```python
from build123d import *

# Parameters (mm, degrees)
SKETCH1_R           = 1.75
SKETCH1_R_2         = 5
BOSS_EXTRUDE1_DEPTH = 6
SKETCH2_R           = 3
SKETCH2_R_2         = 1.75
CUT_EXTRUDE1_DEPTH  = 3
CUT_EXTRUDE2_START  = -3
SKETCH3_R           = 8
SKETCH3_R_2         = 5
CUT_EXTRUDE2_DEPTH  = 3


with BuildPart() as part:
    # Sketch1 → Boss-Extrude1 (new body)
    with BuildSketch(Plane(origin=(0, 0, 0), x_dir=(1, 0, 0), z_dir=(0, 1, 0))):
        with BuildLine():
            Line((23.69, 13.5), (-31.1, 13.5))
            Line((-31.1, 13.5), (-31.1, 10.5))
            ThreePointArc((-31.1, 10.5), (-20.6, 0), (-31.1, -10.5))
            Line((-31.1, -10.5), (-31.1, -13.5))
            Line((-31.1, -13.5), (23.69, -13.5))
            Line((23.69, -13.5), (23.69, -11))
            ThreePointArc((23.69, -11), (34.69, 0), (23.69, 11))
            Line((23.69, 11), (23.69, 13.5))
        make_face()
        with Locations(Location((-12, -9, 0), (0, 0, 270))):
            Circle(SKETCH1_R, mode=Mode.SUBTRACT)
        with Locations(Location((12, -9, 0), (0, 0, 270))):
            Circle(SKETCH1_R, mode=Mode.SUBTRACT)
        with Locations(Location((-12, 9, 0), (0, 0, 270))):
            Circle(SKETCH1_R, mode=Mode.SUBTRACT)
        with Locations(Location((0, 0, 0), (0, 0, 270))):
            Circle(SKETCH1_R_2, mode=Mode.SUBTRACT)
        with Locations(Location((12, 9, 0), (0, 0, 270))):
            Circle(SKETCH1_R, mode=Mode.SUBTRACT)
        with Locations(Location((23.69, 0, 0), (0, 0, 270))):
            Circle(SKETCH1_R_2, mode=Mode.SUBTRACT)
    extrude(amount=BOSS_EXTRUDE1_DEPTH)

    # Sketch2 → Cut-Extrude1 (cut)
    # profile 1 of 4: a face of its own
    with BuildSketch(Plane.XZ):
        with Locations(Location((-12, -9, 0), (0, 0, 270))):
            Circle(SKETCH2_R)
        with Locations(Location((-12, -9, 0), (0, 0, 270))):
            Circle(SKETCH2_R_2, mode=Mode.SUBTRACT)
    # profile 2 of 4: a face of its own
    with BuildSketch(Plane.XZ):
        with Locations(Location((-12, 9, 0), (0, 0, 270))):
            Circle(SKETCH2_R)
        with Locations(Location((-12, 9, 0), (0, 0, 270))):
            Circle(SKETCH2_R_2, mode=Mode.SUBTRACT)
    # profile 3 of 4: a face of its own
    with BuildSketch(Plane.XZ):
        with Locations(Location((12, 9, 0), (0, 0, 270))):
            Circle(SKETCH2_R)
        with Locations(Location((12, 9, 0), (0, 0, 270))):
            Circle(SKETCH2_R_2, mode=Mode.SUBTRACT)
    # profile 4 of 4: a face of its own
    with BuildSketch(Plane.XZ):
        with Locations(Location((12, -9, 0), (0, 0, 270))):
            Circle(SKETCH2_R)
        with Locations(Location((12, -9, 0), (0, 0, 270))):
            Circle(SKETCH2_R_2, mode=Mode.SUBTRACT)
    extrude(amount=-CUT_EXTRUDE1_DEPTH, mode=Mode.SUBTRACT)

    # Sketch3 → Cut-Extrude2 (cut)
    # profile 1 of 2: a face of its own
    with BuildSketch(Plane(origin=(0, 6, 0), x_dir=(1, 0, 0), z_dir=(0, 1, 0)).offset(CUT_EXTRUDE2_START)):
        with Locations(Location((0, 0, 0), (0, 0, 270))):
            Circle(SKETCH3_R)
        with Locations(Location((0, 0, 0), (0, 0, 270))):
            Circle(SKETCH3_R_2, mode=Mode.SUBTRACT)
    # profile 2 of 2: a face of its own
    with BuildSketch(Plane(origin=(0, 6, 0), x_dir=(1, 0, 0), z_dir=(0, 1, 0)).offset(CUT_EXTRUDE2_START)):
        with Locations(Location((23.69, 0, 0), (0, 0, 270))):
            Circle(SKETCH3_R)
        with Locations(Location((23.69, 0, 0), (0, 0, 270))):
            Circle(SKETCH3_R_2, mode=Mode.SUBTRACT)
    extrude(amount=CUT_EXTRUDE2_DEPTH, mode=Mode.SUBTRACT)


solid = part.part
```
CAD build for the part. Positions are in the model's coordinates, mm. A direction names the side the tool comes from. Round coordinates to 2 decimals unless told otherwise and drop trailing zeros. Write each loop counter-clockwise with the first axis right and the second up, starting at its lowest first coordinate (ties: lowest second). Pieces come first, ordered by that corner, then holes.
Item 1: Band-saw the part on D-D on x = -21.5. Write the cut outline in (y, z).
Filled in:
outline: (0, -13.5) - (6, -13.5) - (6, -4.25) - (0, -4.25) - close; (0, 4.25) - (6, 4.25) - (6, 13.5) - (0, 13.5) - close
Item 2: Band-saw the part on A-A on z = 0. Write the cut outline in (x, y).
Filled in:
outline: (-20.6, 0) - (-5, 0) - (-5, 3) - (-8, 3) - (-8, 6) - (-20.6, 6) - close; (5, 0) - (18.69, 0) - (18.69, 3) - (15.69, 3) - (15.69, 6) - (8, 6) - (8, 3) - (5, 3) - close; (28.69, 0) - (34.69, 0) - (34.69, 6) - (31.69, 6) - (31.69, 3) - (28.69, 3) - close
Item 3: Tool access for faces 4 (the flat face through (-5.2, 3, -0.1)), 5 (the flat face through (10, 3, 9)), 6 (the cylindrical face through (-10.5, 4.5, 9.9)), 7 (the flat face through (-31.1, 3, 12)), 8 (the flat face through (23.69, 3, 12)): list every direction of +Z, -Z, +X, -X, +Y, -Y with a clear straight run to the whole face (end or side of a thin tool).
Filled in:
face 4: +Y
face 5: -Y
face 6: +Y, -Y
face 7: +Z, -Z, -X, +Y, -Y
face 8: +Z, +X, +Y, -Y
Item 4: Mould opens along Z. For faces 1 (the flat face through (-3, 3, -13.5)), 2 (the flat face through (23.69, 3, -12)), 3 (the cylindrical face through (-13.15, 1.48, -11.77)) say: released by +Z, released by -Z, zero draft, split by the parting line, or undercut.
Filled in:
face 1: released by -Z
face 2: zero draft
face 3: undercut
Item 5: Band-saw the part on C-C on y = 4.9. Write the cut outline in (x, z), then the cut area to 3 significant figures.
Filled in:
outline: (-31.1, -13.5) - (23.69, -13.5) - (23.69, -11) arc R11 ccw to (23.69, 11) - (23.69, 13.5) - (-31.1, 13.5) - (-31.1, 10.5) arc R10.5 cw to (-31.1, -10.5) - close; hole circle Ø3.5 at (-12, -9); hole circle Ø3.5 at (-12, 9); hole circle Ø16 at (0, 0); hole circle Ø3.5 at (12, -9); hole circle Ø3.5 at (12, 9); hole circle Ø16 at (23.69, 0)
area: 1,060 mm2
Item 6: Drill centre lines: L1, parallel to X at y = 2.2, z = 0; L2, parallel to X at y = 5.05, z = -9; L3, parallel to Z at x = 9.5, y = 2.8. Where is each one in solid material? Low to high.
Filled in:
L1: x = -20.6 to -5, 5 to 18.69, 28.69 to 34.69
L2: x = -25.69 to -13.75, -10.25 to 10.25, 13.75 to 30.01
L3: z = -13.5 to -10.66, -7.34 to 7.34, 10.66 to 13.5
Item 7: Band-saw the part on B-B on x = 12. Write the cut outline in (y, z), then the cut area to 3 significant figures.
Filled in:
outline: (0, -13.5) - (6, -13.5) - (6, -10.75) - (3, -10.75) - (3, -12) - (0, -12) - close; (0, -6) - (3, -6) - (3, -7.25) - (6, -7.25) - (6, 7.25) - (3, 7.25) - (3, 6) - (0, 6) - close; (0, 12) - (3, 12) - (3, 10.75) - (6, 10.75) - (6, 13.5) - (0, 13.5) - close
area: 105 mm2
Item 8: Drop flat-ended pins along their axis: pin 1 Ø6.5 at (x, z) = (-10.5, -10) entering from -Y; pin 2 Ø3 at (x, z) = (-12, -9) entering from -Y; pin 3 Ø1.2 at (y, z) = (4.5, 12.5) entering from +X; pin 4 Ø5.5 at (x, z) = (12, -9) entering from -Y. Give the stop position or say it passes through.
Filled in:
pin 1: stops at y = 0
pin 2: passes through
pin 3: stops at x = 23.69
pin 4: stops at y = 3
